```python
from build123d import *

# Parameters (mm, degrees)
FILLET2_R           = 0.4
SKETCH2_R           = 22.244579061
SKETCH2_R_2         = 21
BOSS_EXTRUDE1_DEPTH = 2
SKETCH3_R           = 21.370804359
SKETCH3_R_2         = 19.170804359
BOSS_EXTRUDE2_DEPTH = 2


with BuildPart() as part:
    # Sketch1 → Revolve1 (revolve)
    with BuildSketch(Plane.XY):
        Polygon((0.662781953, 0), (-8.871246788, 8), (-7.626667727, 8), (1.462781953, 0.373046127), (1.462781953, -0.808290377), (-5.797472085, -5), (-7.997472085, -5), align=None)
    revolve(axis=Axis((13.373332273, 7.609018033, 0), (0, -1, 0)))

    # Fillet2
    fillet2_edges = [part.edges().sort_by_distance(p)[0] for p in [
        (26.083882594, 0, 0),
    ]]
    fillet(fillet2_edges, radius=FILLET2_R)

    # Sketch2 → Boss-Extrude1 (add)
    with BuildSketch(Plane(origin=(0, 8, 0), x_dir=(1, 0, 0), z_dir=(0, 1, 0))):
        with Locations(Location((13.373332273, 0, 0), (0, 0, 180))):
            Circle(SKETCH2_R)
        with Locations(Location((13.373332273, 0, 0), (0, 0, 180))):
            Circle(SKETCH2_R_2, mode=Mode.SUBTRACT)
    extrude(amount=BOSS_EXTRUDE1_DEPTH)

    # Sketch3 → Boss-Extrude2 (add)
    with BuildSketch(Plane.XZ.offset(5)):
        with Locations((13.373332273, 0)):
            Circle(SKETCH3_R)
        with Locations(Location((13.373332273, 0, 0), (0, 0, 180))):
            Circle(SKETCH3_R_2, mode=Mode.SUBTRACT)
    extrude(amount=BOSS_EXTRUDE2_DEPTH)


solid = part.part
```
Read the model definition and answer for the solid it produces. Units are mm, in the model's axes. A direction names the side the tool comes from. Coordinates: 2 decimals unless noted, no trailing zeros. Order: outer loops, then holes, each group sorted by start corner. A loop starts at its lowest first (then second) coordinate and runs counter-clockwise, first axis right, second up. Notation, with made-up numbers: (87.5, 76.5) - (93.5, 76.5) arc R10 ccw to (93.5, 91.5) - close; hole circle Ø1 at (-13.75, 36). An arc over 180 degrees is marked (long way). Answer as a JSON object with one key per item and string values. Group by question number.
Item 1: The mould has two halves that part along Y. Classify faces 1 (the face through (-3, -7, -11)), 2 (the face through (0.29, 0.845, -4.12)), 3 (the face through (3.109, 8.986, -19.735)): +Y half, -Y half, draft (parallel to the pull), parting line (faces both ways), or undercut.
Item 2: Flat-ended cylindrical pins translate along their axes: P1, Ø2, axis at x = 1.5, z = -13.5, coming from the +Y side; P2, Ø25, axis at x = 13.37, z = 0, coming from the -Y side; P3, Ø2, axis at y = 2.5, z = 3.5, coming from the -X side. Find the tip coordinate at first contact, or state that the pin passes through.
Item 3: Consider probe 1 along Y at (x, z) = (33, 0.5); probe 2 along Z at (x, y) = (8, -4.25); probe 3 along Z at (x, y) = (18.5, 2). Determine where each line is inside the solid, lowest interval first. Write a range as from..to.
Item 4: A tool of negligible diameter and unlimited length cuts with its end or side. For faces 4 (the face through (-4.9, -6, -5.8)), 5 (the face through (0.809, -0.515, 5.21)), 6 (the face through (-6.657, 8.986, 6.308)), from which of +Z, -Z, +X, -X, +Y, -Y can it reach the whole face along a straight path? Write none if from no direction.
Item 5: Section B-B (y = -4.25) is taken. Give the vertices of the cut face in (x, z), plus the area to 3 significant figures.
Item 6: Section A-A (y = 3.25) is taken. Give the vertices of the cut face in (x, z).
Results are:
{
 "1": {"face 1": "-Y half", "face 2": "undercut", "face 3": "draft"},
 "2": {"P1": "stops at y = 6.3", "P2": "stops at y = -1.15", "P3": "stops at x = -3.16"},
 "3": {"probe 1": "y = -7..-4, 5.81..6.85", "probe 2": "z = -19.34..-17.04, 17.04..19.34", "probe 3": "z = -14.2..-12.87, 12.87..14.2"},
 "4": {"face 4": "-Y", "face 5": "none", "face 6": "+Y"},
 "5": {"outline": "circle Ø40.14 at (13.37, 0); hole circle Ø35.74 at (13.37, 0)", "area": "262 mm^2"},
 "6": {"outline": "circle Ø33.17 at (13.37, 0); hole circle Ø30.68 at (13.37, 0)"}
}
